from build123d import *

# Parameters (mm, degrees)
F4_D = 6.35


with BuildPart() as f1:
    # F0 (on Front) → F1 (revolve)
    with BuildSketch(Plane.XZ):
        Polygon((-6.985, -88.9), (0, -88.9), (0, 107.95), (-9.398, 107.95), (-9.398, 95.25), (-15.621, 95.25), (-15.621, 88.9), (-9.398, 88.9), (-9.398, -83.82), align=None)
    revolve(axis=Axis((0, 0, 2.568085), (0, 0, -1)))

    # F4 (through all)
    with Locations(Plane.YZ.offset(25.4)):
        with Locations((0, 101.6)):
            Hole(F4_D / 2)

    # F5 (on Front) → F6 (revolve, cut)
    with BuildSketch(Plane.XZ):
        Polygon((-9.398, -69.977), (-9.398, -74.93), (9.398, -74.93), (9.398, -69.977), (8.128, -71.755), (-8.128, -71.755), align=None)
    revolve(axis=Axis((3.955706, 0, -74.93), (1, 0, 0)), mode=Mode.SUBTRACT)


solid = f1.part
Here's how the part is built. I have some questions about the finished solid (model axes, mm). A direction names the side the tool comes from. Coordinates: 2 decimals unless noted, no trailing zeros. Write each loop counter-clockwise with the first axis right and the second up, starting at its lowest first coordinate (ties: lowest second). Pieces come first, ordered by that corner, then holes.
1) Which directions (+Z, -Z, +X, -X, +Y, -Y) give clear straight access to the entire face, cutting with the end or side of a thin tool? Please do faces 1 (the face through (-0.13, -1.707, 104.277)), 2 (the face through (9.39, 0.41, 1.33)), 3 (the face through (-8.68, -3.6, 101.51)).
Filled in:
face 1: +X, -X
face 2: -Z
face 3: +Z
2) If we section it at B-B (x = 0): List the corners of the cut face in (y, z) for me (3 decimals), plus the area to 3 significant figures.
Filled in:
outline: (-15.621, 88.9) - (-9.398, 88.9) - (-9.398, -83.82) - (-6.985, -88.9) - (6.985, -88.9) - (9.398, -83.82) - (9.398, 88.9) - (15.621, 88.9) - (15.621, 95.25) - (9.398, 95.25) - (9.398, 107.95) - (-9.398, 107.95) - (-9.398, 95.25) - (-15.621, 95.25) - close; hole circle Ø6.35 at (0, -74.93); hole circle Ø6.35 at (0, 101.6)
area: 3,700 mm2
3) I'm going to push flat-ended pins straight in: pin 1 (1 mm diameter, centred on y = -5.5, z = 66.5, fed in from +X); pin 2 (3 mm diameter, centred on y = 4.5, z = 58, fed in from +X); pin 3 (1.5 mm diameter, centred on x = -11.5, z = -17, fed in from -Y); pin 4 (1.5 mm diameter, centred on x = -9, y = -3, fed in from -Z). Where does each tip first touch, or does it pass through?
Filled in:
pin 1: stops at x = 7.96
pin 2: stops at x = 8.91
pin 3: passes through
pin 4: stops at z = -85.21
4) Thinking about a two-plate mould opening in Z: for faces 4 (the face through (2.03, 15.49, 92.03)), 5 (the face through (-7, -7, 88.9)), 6 (the face through (-0.11, -0.14, -78.1)), which applies, +Z half, -Z half, draft (parallel to the pull), parting line (faces both ways), or undercut?
Filled in:
face 4: draft
face 5: -Z half
face 6: undercut
5) If we section it at D-D (z = -42): List the corners of the cut face in (x, y) for me, plus the area to 3 significant figures.
Filled in:
outline: circle Ø18.8 at (0, 0)
area: 277 mm2
6) If we section it at C-C (z = -74.93): List the corners of the cut face in (x, y) for me (3 decimals), plus the area to 3 significant figures.
Filled in:
outline: (-8.587, -3.818) arc R9.398 ccw to (8.587, -3.818) - (8.128, -3.175) - (-8.128, -3.175) - close; (-8.587, 3.818) - (-8.128, 3.175) - (8.128, 3.175) - (8.587, 3.818) arc R9.398 ccw to start
area: 159 mm2
7) If I drill on line 1 (Z direction, x = -3, y = 0) (3 decimals); line 2 (Z direction, x = 9.5, y = -2); line 3 (Z direction, x = 9, y = 1), over which ranges is the centre line in solid material (lowest first)?
Filled in:
line 1: z = -88.9 to -78.105, -71.755 to 98.425, 104.775 to 107.95
line 2: z = 88.9 to 95.25
line 3: z = -84.54 to -79.21, -70.65 to 98.59, 104.61 to 107.95
8) If we section it at A-A (y = 0): List the corners of the cut face in (x, z) for me (3 decimals).
Filled in:
outline: (-15.621, 88.9) - (-9.398, 88.9) - (-9.398, -69.977) - (-8.128, -71.755) - (8.128, -71.755) - (9.398, -69.977) - (9.398, 88.9) - (15.621, 88.9) - (15.621, 95.25) - (9.398, 95.25) - (9.398, 98.425) - (-9.398, 98.425) - (-9.398, 95.25) - (-15.621, 95.25) - close; (-9.398, -83.82) - (-6.985, -88.9) - (6.985, -88.9) - (9.398, -83.82) - (9.398, -79.883) - (8.128, -78.105) - (-8.128, -78.105) - (-9.398, -79.883) - close; (-9.398, 104.775) - (9.398, 104.775) - (9.398, 107.95) - (-9.398, 107.95) - close
